from build123d import *

# Parameters (mm, degrees)
SKETCH_1_R           = 1.7
SKETCH_1_R_2         = 5.4
EXTRUDE_1_DEPTH      = 10
EXTRUDE_START        = -10
EXTRUDE_2_DEPTH      = 10
CUT_EXTRUDE_1_DEPTH  = 2
EXTRUDE_START_2      = -46
EXTRUDE_3_DEPTH      = 36
EXTRUDE_START_3      = 6.5
EXTRUDE_4_DEPTH      = 3.5
EXTRUDE_5_DEPTH      = 4
SKETCH_1_10_W        = 8
SKETCH_1_10_H        = 8
SKETCH_1_10_R        = 1.5
EXTRUDE_6_DEPTH      = 7
RIB_2_REACH          = 105.331
SKETCH_4_WALL_W      = 219.975267576
SKETCH_4_WALL_H      = 1
RIB_START            = -1
RIB_3_DEPTH          = 1
EXTRUDE_START_4      = -0.4
SKETCH_6_R           = 1.5
EXTRUDE_7_DEPTH      = 0.4
SKETCH_7_R           = 1.7
SKETCH_7_R_2         = 1.35
CUT_EXTRUDE_2_DEPTH  = 89.290712988
SKETCH_8_W           = 26
SKETCH_8_H           = 10
CUT_EXTRUDE_3_DEPTH  = 105.174133066
CUT_EXTRUDE_4_DEPTH  = 22
CUT_EXTRUDE_5_DEPTH  = 24
SKETCH_7_4_W         = 2.4
SKETCH_7_4_H         = 10
CUT_EXTRUDE_9_DEPTH  = 15.05
CHAMFER_1_SIZE       = 3.7
CUT_EXTRUDE_START    = -17.562916
SKETCH_7_5_W         = 3
SKETCH_7_5_H         = 6
CUT_EXTRUDE_10_DEPTH = 17.562916
CUT_EXTRUDE_11_REACH = 90.291
CHAMFER_2_SIZE       = 5
CHAMFER_3_SIZE       = 2
CHAMFER_3_SIZE2      = 2.5
SKETCH_9_W           = 11.322924712
SKETCH_9_H           = 24.282583949
CUT_EXTRUDE_12_DEPTH = 93.82914413
CUT_EXTRUDE_START_2  = -49
SKETCH_1_14_R        = 1.5
CUT_EXTRUDE_13_DEPTH = 10


# Read off the part's stored shape, not the designer's step: 筋3
with BuildPart() as part:
    # 草图1 → 凸台-拉伸1 (new body)
    with BuildSketch(Plane.XY):
        with BuildLine():
            Line((-17, -7.5), (-17, -11))
            Line((-17, -11), (0, -11))
            ThreePointArc((0, -11), (7.778174593, -7.778174593), (11, 0))
            Line((11, 0), (11, 8.456854249))
            Line((11, 8.456854249), (28, 8.456854249))
            Line((28, 8.456854249), (28, 10.5))
            Line((28, 10.5), (21, 10.5))
            Line((21, 10.5), (21, 20.5))
            Line((21, 20.5), (28, 20.5))
            Line((28, 20.5), (28, 23.5))
            Line((28, 23.5), (-67, 23.5))
            Line((-67, 23.5), (-67, 7.5))
            Line((-67, 7.5), (-17, 7.5))
            ThreePointArc((-17, 7.5), (-9.5, 0), (-17, -7.5))
        make_face()
        with Locations((-5.656854249, -5.656854249)):
            Circle(SKETCH_1_R, mode=Mode.SUBTRACT)
        with Locations((5.656854249, -5.656854249)):
            Circle(SKETCH_1_R, mode=Mode.SUBTRACT)
        Circle(SKETCH_1_R_2, mode=Mode.SUBTRACT)
        with Locations((-5.656854249, 5.656854249)):
            Circle(SKETCH_1_R, mode=Mode.SUBTRACT)
        with Locations((5.656854249, 5.656854249)):
            Circle(SKETCH_1_R, mode=Mode.SUBTRACT)
    extrude(amount=EXTRUDE_1_DEPTH)

    # 草图1<6> → 凸台-拉伸2 (add)
    with BuildSketch(Plane.XY.offset(EXTRUDE_START)):
        with BuildLine():
            Line((21, 10.5), (21, 20.5))
            Line((21, 20.5), (28, 20.5))
            Line((28, 20.5), (28, 23.5))
            Line((28, 23.5), (-67, 23.5))
            Line((-67, 23.5), (-67, 7.5))
            Line((-67, 7.5), (-17, 7.5))
            ThreePointArc((-17, 7.5), (-9.5, 0), (-17, -7.5))
            Line((-17, -7.5), (-17, -11))
            ThreePointArc((-17, -11), (-8.462447466, -5.036106671), (-8.643737412, 5.376624039))
            ThreePointArc((-8.643737412, 5.376624039), (-7.46899014, 8.047704206), (-4.579821288, 8.456854249))
            Line((-4.579821288, 8.456854249), (28, 8.456854249))
            Line((28, 8.456854249), (28, 10.5))
            Line((28, 10.5), (21, 10.5))
        make_face()
    extrude(amount=EXTRUDE_2_DEPTH)

    # 草图3 → 切除-拉伸1 (cut)
    with BuildSketch(Plane(origin=(0, 0, 0), x_dir=(-1, 0, 0), z_dir=(0, 0, -1))):
        Polygon((7.919595949, 3.39411255), (8.747816894, 6.485075194), (6.485075194, 8.747816894), (3.39411255, 7.919595949), (2.565891605, 4.828633305), (4.828633305, 2.565891605), align=None)
        Polygon((-2.565891605, 4.828633305), (-3.39411255, 7.919595949), (-6.485075194, 8.747816894), (-8.747816894, 6.485075194), (-7.919595949, 3.39411255), (-4.828633305, 2.565891605), align=None)
        Polygon((-3.39411255, -7.919595949), (-2.565891605, -4.828633305), (-4.828633305, -2.565891605), (-7.919595949, -3.39411255), (-8.747816894, -6.485075194), (-6.485075194, -8.747816894), align=None)
        Polygon((2.565891605, -4.828633305), (3.39411255, -7.919595949), (6.485075194, -8.747816894), (8.747816894, -6.485075194), (7.919595949, -3.39411255), (4.828633305, -2.565891605), align=None)
    extrude(amount=-CUT_EXTRUDE_1_DEPTH, mode=Mode.SUBTRACT)

    # 草图1<7> → 凸台-拉伸3 (add)
    with BuildSketch(Plane.XY.offset(EXTRUDE_START_2)):
        with BuildLine():
            Line((21, 8.456854249), (21, 23.5))
            Line((21, 23.5), (-67, 23.5))
            Line((-67, 23.5), (-67, 7.5))
            Line((-67, 7.5), (-17, 7.5))
            ThreePointArc((-17, 7.5), (-9.5, 0), (-17, -7.5))
            Line((-17, -7.5), (-17, -11))
            ThreePointArc((-17, -11), (-8.462447466, -5.036106671), (-8.643737412, 5.376624039))
            ThreePointArc((-8.643737412, 5.376624039), (-7.46899014, 8.047704206), (-4.579821288, 8.456854249))
            Line((-4.579821288, 8.456854249), (21, 8.456854249))
        make_face()
    extrude(amount=EXTRUDE_3_DEPTH)

    # 草图1<8> → 凸台-拉伸4 (add)
    with BuildSketch(Plane.XY.offset(EXTRUDE_START_3)):
        with BuildLine():
            Line((-17, -5), (-17, -7.5))
            ThreePointArc((-17, -7.5), (-9.5, 0), (-17, 7.5))
            Line((-17, 7.5), (-17, 5))
            ThreePointArc((-17, 5), (-12, 0), (-17, -5))
        make_face()
    extrude(amount=EXTRUDE_4_DEPTH)

    # 草图1<9> → 凸台-拉伸5 (add)
    with BuildSketch(Plane.XY.offset(EXTRUDE_START_2)):
        with BuildLine():
            Line((-17, -5), (-17, -7.5))
            ThreePointArc((-17, -7.5), (-9.5, 0), (-17, 7.5))
            Line((-17, 7.5), (-17, 5))
            ThreePointArc((-17, 5), (-12, 0), (-17, -5))
        make_face()
    extrude(amount=EXTRUDE_5_DEPTH)

    # 草图1<10> → 凸台-拉伸6 (add)
    with BuildSketch(Plane.XY.offset(EXTRUDE_START_2)):
        with Locations((16, 27.5)):
            Rectangle(SKETCH_1_10_W, SKETCH_1_10_H)
        with Locations((16, 27.5)):
            Circle(SKETCH_1_10_R, mode=Mode.SUBTRACT)
    extrude(amount=EXTRUDE_6_DEPTH)

    # 草图4 wall → 筋2 (add, up to next)
    with BuildSketch(Plane(origin=(20, 27.5, -35), x_dir=(0, -0.707106781187, 0.707106781187), z_dir=(0, -0.707106781187, -0.707106781187)), mode=Mode.PRIVATE) as rib_2_sk1:
        with Locations((0, 0.5)):
            Rectangle(SKETCH_4_WALL_W, SKETCH_4_WALL_H)
    rib_2_tool1 = extrude(rib_2_sk1.sketch, amount=RIB_2_REACH, mode=Mode.PRIVATE) - part.part
    add(rib_2_tool1.solids().sort_by_distance((20, 27.5, -35))[0])

    # 筋3 outline → 筋3 (add)
    with BuildSketch(Plane.ZY.offset(-12).offset(RIB_START)):
        Polygon((-31, 23.5), (-39, 31.5), (-39, 23.5), align=None)
    extrude(amount=RIB_3_DEPTH)

    # 草图6 → 凸台-拉伸7 (add)
    with BuildSketch(Plane.XY.offset(-39).offset(EXTRUDE_START_4)):
        with Locations((16, 27.5)):
            Circle(SKETCH_6_R)
    extrude(amount=EXTRUDE_7_DEPTH)

    # 草图7 → 切除-拉伸2 (cut, through all)
    with BuildSketch(Plane(origin=(0, 23.5, 0), x_dir=(1, 0, 0), z_dir=(0, 1, 0))):
        with BuildLine():
            Line((-17, 38), (-17, 46))
            Line((-17, 46), (-69, 46))
            Line((-69, 46), (-69, 5))
            Line((-69, 5), (-48, 5))
            ThreePointArc((-48, 5), (-38.807611845, 8.807611845), (-35, 18))
            Line((-35, 18), (-35, 38))
            Line((-35, 38), (-17, 38))
        make_face()
        with Locations(Location((12.7, 18, 0), (0, 0, 180))):
            Circle(SKETCH_7_R)
        with Locations(Location((16, -6, 0), (0, 0, 180))):
            Circle(SKETCH_7_R)
        with Locations(Location((8, 42, 0), (0, 0, 180))):
            Circle(SKETCH_7_R)
        with Locations(Location((-32.5, 2.5, 0), (0, 0, 180))):
            Circle(SKETCH_7_R)
        with Locations(Location((-63.5, 2.5, 0), (0, 0, 180))):
            Circle(SKETCH_7_R)
        with Locations(Location((-32.5, 33.5, 0), (0, 0, 180))):
            Circle(SKETCH_7_R)
        with Locations(Location((24.5, -5, 0), (0, 0, 180))):
            Circle(SKETCH_7_R_2)
        with Locations(Location((24.5, 5, 0), (0, 0, 270))):
            Circle(SKETCH_7_R_2)
    extrude(amount=-CUT_EXTRUDE_2_DEPTH, mode=Mode.SUBTRACT)

    # 草图8 → 切除-拉伸3 (cut, through all)
    with BuildSketch(Plane(origin=(21, 0, 0), x_dir=(0, 0, -1), z_dir=(1, 0, 0))):
        with Locations((18, 15.5)):
            Rectangle(SKETCH_8_W, SKETCH_8_H)
    extrude(amount=-CUT_EXTRUDE_3_DEPTH, mode=Mode.SUBTRACT)

    # 草图8<3> → 切除-拉伸4 (cut)
    with BuildSketch(Plane(origin=(21, 0, 0), x_dir=(0, 0, -1), z_dir=(1, 0, 0))):
        with BuildLine():
            ThreePointArc((36, 19.7), (31.8, 15.5), (36, 11.3))
            Line((36, 11.3), (36, 19.7))
        make_face()
        with BuildLine():
            ThreePointArc((4.2, 15.5), (2.969848481, 18.469848481), (0, 19.7))
            Line((0, 19.7), (0, 11.3))
            ThreePointArc((0, 11.3), (2.969848481, 12.530151519), (4.2, 15.5))
        make_face()
    extrude(amount=-CUT_EXTRUDE_4_DEPTH, mode=Mode.SUBTRACT)

    # 草图8<4> → 切除-拉伸5 (cut)
    with BuildSketch(Plane(origin=(21, 0, 0), x_dir=(0, 0, -1), z_dir=(1, 0, 0))):
        with BuildLine():
            Line((0, 11.3), (0, 19.7))
            ThreePointArc((0, 19.7), (-2.787471973, 18.641655614), (-4.170131892, 16))
            Line((-4.170131892, 16), (-10, 16))
            Line((-10, 16), (-10, 15))
            Line((-10, 15), (-4.170131892, 15))
            ThreePointArc((-4.170131892, 15), (-2.787471973, 12.358344386), (0, 11.3))
        make_face()
        with BuildLine():
            Line((40.170131892, 15), (46, 15))
            Line((46, 15), (46, 16))
            Line((46, 16), (40.170131892, 16))
            ThreePointArc((40.170131892, 16), (38.787471973, 18.641655614), (36, 19.7))
            Line((36, 19.7), (36, 11.3))
            ThreePointArc((36, 11.3), (38.787471973, 12.358344386), (40.170131892, 15))
        make_face()
    extrude(amount=-CUT_EXTRUDE_5_DEPTH, mode=Mode.SUBTRACT)

    # 草图7<4> → 切除-拉伸9 (cut)
    with BuildSketch(Plane(origin=(0, 23.5, 0), x_dir=(1, 0, 0), z_dir=(0, 1, 0))):
        with Locations((-2.2, -5)):
            Rectangle(SKETCH_7_4_W, SKETCH_7_4_H)
        with Locations((-2.2, 41)):
            Rectangle(SKETCH_7_4_W, SKETCH_7_4_H)
    extrude(amount=-CUT_EXTRUDE_9_DEPTH, mode=Mode.SUBTRACT)

    # 倒角1
    chamfer_1_edges = [part.edges().sort_by_distance(p)[0] for p in [
        (-1, 16, -43.085065946),
        (-1, 15, -43.085065946),
        (-1, 16, 7.085065946),
        (-1, 15, 7.085065946),
    ]]
    chamfer(chamfer_1_edges, length=CHAMFER_1_SIZE)

    # 草图7<5> → 切除-拉伸10 (cut)
    with BuildSketch(Plane(origin=(0, 23.5, 0), x_dir=(1, 0, 0), z_dir=(0, 1, 0)).offset(CUT_EXTRUDE_START)):
        with Locations((-7.143737412, 18)):
            Rectangle(SKETCH_7_5_W, SKETCH_7_5_H)
        with Locations((-7.143737412, 28)):
            Rectangle(SKETCH_7_5_W, SKETCH_7_5_H)
        with Locations((-23, 28)):
            Rectangle(SKETCH_7_5_W, SKETCH_7_5_H)
        with Locations((-23, 18)):
            Rectangle(SKETCH_7_5_W, SKETCH_7_5_H)
        with Locations((-23, 8)):
            Rectangle(SKETCH_7_5_W, SKETCH_7_5_H)
        with Locations((-7.143737412, 8)):
            Rectangle(SKETCH_7_5_W, SKETCH_7_5_H)
    extrude(amount=CUT_EXTRUDE_10_DEPTH, mode=Mode.SUBTRACT)

    # 草图7<6> → 切除-拉伸11 (cut, up to next)
    with BuildSketch(Plane(origin=(0, 23.5, 0), x_dir=(1, 0, 0), z_dir=(0, 1, 0)), mode=Mode.PRIVATE) as cut_extrude_11_sk1:
        Polygon((-21.5, 5), (-8.643737412, 5), (-8.643737412, 11), (-5.643737412, 11), (-5.643737412, 15), (-8.643737412, 15), (-8.643737412, 21), (-5.643737412, 21), (-5.643737412, 25), (-8.643737412, 25), (-8.643737412, 31), (-21.5, 31), (-21.5, 25), (-24.5, 25), (-24.5, 21), (-21.5, 21), (-21.5, 15), (-24.5, 15), (-24.5, 11), (-21.5, 11), align=None)
    cut_extrude_11_tool1 = extrude(cut_extrude_11_sk1.sketch, amount=-CUT_EXTRUDE_11_REACH, mode=Mode.PRIVATE) & part.part
    add(cut_extrude_11_tool1.solids().sort_by_distance((-15.071869, 23.5, -18))[0], mode=Mode.SUBTRACT)

    # 倒角2
    chamfer_2_edges = [part.edges().sort_by_distance(p)[0] for p in [
        (-5.643737412, 22, -31),
        (-24.5, 22, -31),
    ]]
    chamfer(chamfer_2_edges, length=CHAMFER_2_SIZE)

    # 倒角3
    chamfer_3_edges = [part.edges().sort_by_distance(p)[0] for p in [
        (-12, 0, -42),
    ]]
    chamfer_3_side = [part.faces().sort_by_distance(p)[0] for p in [
        (-9.667705098, 0, -42),
    ]]
    chamfer(chamfer_3_edges, length=CHAMFER_3_SIZE, length2=CHAMFER_3_SIZE2, reference=chamfer_3_side[0])

    # 草图9 → 切除-拉伸12 (cut, through all)
    with BuildSketch(Plane.XY.offset(10)):
        with Locations((25.661462356, 19.358708026)):
            Rectangle(SKETCH_9_W, SKETCH_9_H)
    extrude(amount=-CUT_EXTRUDE_12_DEPTH, mode=Mode.SUBTRACT)

    # 草图1<14> → 切除-拉伸13 (cut)
    with BuildSketch(Plane.XY.offset(CUT_EXTRUDE_START_2)):
        with Locations((16, 27.5)):
            Circle(SKETCH_1_14_R)
    extrude(amount=CUT_EXTRUDE_13_DEPTH, mode=Mode.SUBTRACT)


solid = part.part
Check sheet for the modelled part. Datum: model origin and axes. Units: mm. A direction names the side the tool comes from. Round coordinates to 2 decimals unless told otherwise and drop trailing zeros. Order: outer loops, then holes, each group sorted by start corner. A loop starts at its lowest first (then second) coordinate and runs counter-clockwise, first axis right, second up.
Q1. Draft check along Y on faces 4 (the face through (-24, 14, 10)), 5 (the face through (14.89, 28.51, -42.55)), 6 (the face through (-2, 8.45, 5)), 7 (the face through (-2.974, -6.352, 0.986)). Enter one of: pulls with the +Y half, pulls with the -Y half, needs draft (parallel to the pull), parting line crosses it, or undercut.
Filled sheet:
face 4: needs draft
face 5: undercut
face 6: pulls with the +Y half
face 7: undercut
Q2. Depth check by flat-ended pin: P1, Ø4, axis at x = -13.5, y = -2, coming from the -Z side; P2, Ø4, axis at x = 8, z = -42, coming from the -Y side; P3, Ø3, axis at x = -18, z = -9.5, coming from the -Y side; P4, Ø1.5, axis at y = 9.5, z = -28, coming from the -X side. Enter the tip coordinate at first touch or a pass-through.
Filled sheet:
P1: stops at z = -46
P2: stops at y = 8.46
P3: stops at y = -11
P4: stops at x = -35
Q3. Cross-section at A-A, the plane y = 13.5. Give the number of separate pieces and of enclosed holes in the cut face, plus the area to 3 significant figures.
Filled sheet:
separate pieces: 4
enclosed holes: 5
area: 1,550 mm2
Q4. Cross-section at D-D, the plane z = -2.5. Enter the section's corners in (x, y).
Filled sheet:
outline: (-67, 7.5) - (-65.2, 7.5) - (-65.2, 23.5) - (-67, 23.5) - close; (-61.8, 7.5) - (-34.2, 7.5) - (-34.2, 23.5) - (-61.8, 23.5) - close; (-30.8, 7.5) - (-17, 7.5) arc R7.5 cw to (-17, -7.5) - (-17, -11) arc R11.08 ccw to (-8.64, 5.38) arc R3 cw to (-4.58, 8.46) - (20, 8.46) - (20, 12.13) - (-1, 12.13) - (-1, 18.87) - (20, 18.87) - (20, 23.5) - (-30.8, 23.5) - close
Q5. Scan lines: L1, parallel to Y at x = 3.5, z = -23; L2, parallel to Z at x = -32, y = 17; L3, parallel to Z at x = -18.5, y = 14.5. Record each from-to range of solid material in increasing order.
Filled sheet:
L1: y = 8.46 to 10.5, 20.5 to 23.5
L2: z = -38 to -35.12, -31.88 to -31, -5 to -4.12, -0.88 to 10
L3: z = -38 to -31, -5 to 10
Q6. Set-up check for faces 1 (the face through (6.352, -2.974, 0.986)), 2 (the face through (-8.644, 8, -8)), 3 (the face through (-7.632, 7.601, 0.986)): record each of +Z, -Z, +X, -X, +Y, -Y from which the full face is reachable in a straight line by a thin tool's end or side.
Filled sheet:
face 1: -Z
face 2: +Y
face 3: none
Q7. Cross-section at C-C, the plane y = 27.5. Enter the section's corners in (x, z).
Filled sheet:
outline: (12, -46) - (14.5, -46) - (14.5, -39) - (13, -39) - (13, -35) - (12, -35) - close; (17.5, -46) - (20, -46) - (20, -35) - (19, -35) - (19, -39) - (17.5, -39) - close
Q8. Cross-section at B-B, the plane x = -22.5. Enter the section's corners in (y, z).
Filled sheet:
outline: (7.5, -38) - (23.5, -38) - (23.5, -28) - (20.5, -28) - (20.5, -31) - (7.5, -31) - close; (7.5, -25) - (10.5, -25) - (10.5, -21) - (7.5, -21) - close; (7.5, -15) - (10.5, -15) - (10.5, -11) - (7.5, -11) - close; (7.5, -5) - (23.5, -5) - (23.5, 10) - (7.5, 10) - close
